from build123d import *

# Parameters (mm, degrees)
PAD_DEPTH       = 16
SKETCH_R        = 4
POCKET_DEPTH    = 632.001
SKETCH002_R     = 4
POCKET001_DEPTH = 400.001
SKETCH003_R     = 4
POCKET002_DEPTH = 16.001
SKETCH004_R     = 4
POCKET003_DEPTH = 16.001


with BuildPart() as part:
    # Sketch001 → Pad (new body)
    with BuildSketch(Plane.XZ):
        Polygon((300, 0), (300, -100), (316, -100), (316, 300), (-316, 300), (-316, -100), (-300, -100), (-300, 0), (-300, 284), (300, 284), align=None)
    extrude(amount=PAD_DEPTH)

    # Sketch (on Face4 of Pad) → Pocket (cut, through all)
    with BuildSketch(Plane(origin=(-316, 0, 0), x_dir=(0, 0, -1), z_dir=(-1, 0, 0))):
        with Locations((0, 8)):
            Circle(SKETCH_R)
    extrude(amount=-POCKET_DEPTH, mode=Mode.SUBTRACT)

    # Sketch002 (on Face8 of Pocket) → Pocket001 (cut, through all)
    with BuildSketch(Plane(origin=(0, 0, 300), x_dir=(-1, 0, 0), z_dir=(0, 0, 1))):
        with Locations((-50, 8)):
            Circle(SKETCH002_R)
        with Locations((50, 8)):
            Circle(SKETCH002_R)
    extrude(amount=-POCKET001_DEPTH, mode=Mode.SUBTRACT)

    # Sketch003 (on Face4 of Pocket001) → Pocket002 (cut, through all)
    with BuildSketch(Plane(origin=(0, 0, 0), x_dir=(1, 0, 0), z_dir=(0, 1, 0))):
        with Locations((308, -50)):
            Circle(SKETCH003_R)
        with Locations((-308, -50)):
            Circle(SKETCH003_R)
    extrude(amount=-POCKET002_DEPTH, mode=Mode.SUBTRACT)

    # Sketch004 (on Face4 of Pocket002) → Pocket003 (cut, through all)
    with BuildSketch(Plane(origin=(0, 0, 0), x_dir=(1, 0, 0), z_dir=(0, 1, 0))):
        with Locations((308, -160)):
            Circle(SKETCH004_R)
        with Locations((-308, -160)):
            Circle(SKETCH004_R)
    extrude(amount=-POCKET003_DEPTH, mode=Mode.SUBTRACT)


solid = part.part
Geometry: final body of the model. Coordinates: model frame, mm. A direction names the side the tool comes from. Give positions to 0.01 mm unless a question says otherwise; leave off trailing zeros. Loops run counter-clockwise (first coordinate to the right, second up) from the corner with the lowest first, then second, coordinate; pieces in that order, holes last. Notation, with made-up numbers: M 0.5,14.5 L 48.5,14.5 A21 cw 48.5,23.5 Z; hole C 41,47 d1. An arc over 180 degrees is marked long. Put each result on its own line as item: value.
1) Mould query, pull axis X, two halves, no side actions, for faces 3 (the flat face through (316, -8, 97)), 4 (the flat face through (-1, 0, 294)), 5 (the flat face through (-300, -8, 89)). Classes: released by +X, released by -X, zero draft, split by the parting line, or undercut.
Computed values:
face 3: released by +X
face 4: zero draft
face 5: undercut
2) Cut plane B-B, the plane y = -8. Give the number of separate pieces and of enclosed holes in the cut face, plus the area to 3 significant figures.
Computed values:
separate pieces: 5
enclosed holes: 4
area: 21,700 mm^2
3) Cut plane A-A, the plane z = 21.5. Return the cut outline in (x, y).
Computed values:
outline: M -316,-16 L -300,-16 L -300,0 L -316,0 Z; M 300,-16 L 316,-16 L 316,0 L 300,0 Z
4) Reachability of faces 1 (the flat face through (-308, -8, -100)), 2 (the flat face through (300, -8, 95)) from +Z, -Z, +X, -X, +Y, -Y: full face, straight path, thin tool, end or side. Return the list, or none.
Computed values:
face 1: -Z, +X, -X, +Y, -Y
face 2: -Z, +Y, -Y
5) First-contact query: P1, Ø9, axis at x = 50, y = -8, coming from the -Z side; P2, Ø7, axis at y = -8, z = 0, coming from the -X side; P3, Ø10.5, axis at x = -308, z = 160, coming from the +Y side. Flat tips, straight axial feed; report the tip coordinate or a pass-through.
Computed values:
P1: stops at z = 284
P2: passes through
P3: stops at y = 0
6) Cut plane C-C, the plane x = -154.5. Return the cut outline in (y, z).
Computed values:
outline: M -16,284 L 0,284 L 0,300 L -16,300 Z
7) Material intervals for L1, parallel to X at y = -8, z = 289; L2, parallel to X at y = -8, z = 50; L3, parallel to Z at x = 308, y = -8.5, sorted ascending. Write a range as from..to.
Computed values:
L1: x = -316..-54, -46..46, 54..316
L2: x = -316..-312, -304..-300, 300..304, 312..316
L3: z = -100..-3.97, 3.97..46, 54..156, 164..300
